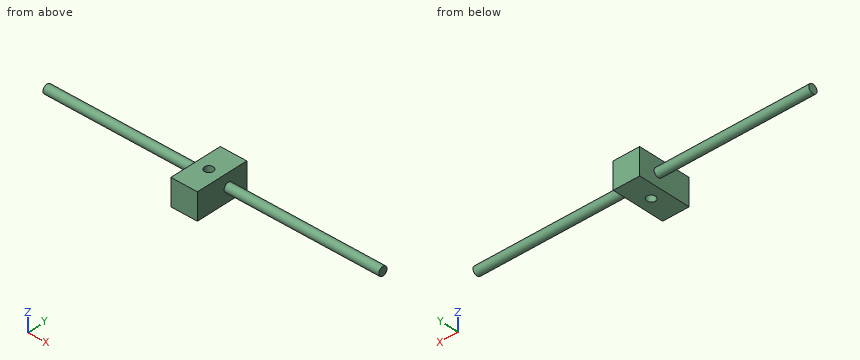
from build123d import *

# Parameters (mm, degrees)
SKETCH_1_W      = 60
SKETCH_1_H      = 120
SKETCH_1_R      = 10
EXTRUDE_1_DEPTH = 30
SKETCH_2_R      = 10
EXTRUDE_2_DEPTH = 350
EXTRUDE_START   = 350
SKETCH_3_R      = 10
EXTRUDE_3_DEPTH = 350


with BuildPart() as part:
    # Эскиз1 → Бобышка-Вытянуть1 (new, symmetric)
    with BuildSketch(Plane.XY):
        Rectangle(SKETCH_1_W, SKETCH_1_H)
        with Locations(Location((0, 0, 0), (0, 0, 180))):
            Circle(SKETCH_1_R, mode=Mode.SUBTRACT)
    extrude(amount=EXTRUDE_1_DEPTH, both=True)

    # Эскиз2 → Бобышка-Вытянуть2 (add)
    with BuildSketch(Plane.ZY.offset(30)):
        with Locations(Location((0, 15, 0), (0, 0, 270))):
            Circle(SKETCH_2_R)
    extrude(amount=EXTRUDE_2_DEPTH)

    # Эскиз3 → Бобышка-Вытянуть3 (add)
    with BuildSketch(Plane(origin=(30, 0, 0), x_dir=(0, 0, -1), z_dir=(1, 0, 0)).offset(EXTRUDE_START)):
        with Locations(Location((0, 15, 0), (0, 0, 270))):
            Circle(SKETCH_3_R)
    extrude(amount=-EXTRUDE_3_DEPTH)


solid = part.part
Can you work these out from the model? Positions are in its coordinate system, mm. Coordinates: 2 decimals unless noted, no trailing zeros. Loops run counter-clockwise (first coordinate to the right, second up) from the corner with the lowest first, then second, coordinate; pieces in that order, holes last. Notation, with made-up numbers: M -40,75.5 L -7,75.5 A23 cw -7,102.5 Z; hole C 14,65 d2. An arc over 180 degrees is marked long. Answer as CSV lines item,"result". Start each with the question number.
1. Suppose I cut it at B-B, the plane x = 0. List the corners of the cut face in (y, z) for me, plus the area to 3 significant figures.
2. Suppose I cut it at C-C, the plane y = -35. List the corners of the cut face in (x, z) for me, plus the area to 3 significant figures.
3. For pin 1 Ø1 at (x, z) = (95, 7.5) entering from -Y; pin 2 Ø10 at (x, z) = (-106.5, -3.5) entering from -Y; pin 3 Ø1.5 at (y, z) = (-15.5, -17) entering from -X, each with a flat end and sliding along its axis, tell me the tip position at first contact or that it passes through.
4. If I drill on probe 1 along Y at (x, z) = (0, -16); probe 2 along X at (y, z) = (49.5, 23); probe 3 along X at (y, z) = (7, -8), over which ranges is the centre line in solid material (lowest first)? Write a range as [from, to].
5. Suppose I cut it at A-A, the plane z = 20.5. List the corners of the cut face in (x, y) for me, plus the area to 3 significant figures.
6. Suppose I cut it at D-D, the plane x = -263.5. List the corners of the cut face in (y, z) for me.
Output:
1,outline,"M -60,-30 L -10,-30 L -10,30 L -60,30 Z; M 10,-30 L 60,-30 L 60,30 L 10,30 Z"
1,area,"6,000 mm^2"
2,outline,"M -30,-30 L 30,-30 L 30,30 L -30,30 Z"
2,area,"3,600 mm^2"
3,pin 1,"stops at y = 7.86"
3,pin 2,"stops at y = 5"
3,pin 3,"stops at x = -30"
4,probe 1,"y = [-60, -10], [10, 60]"
4,probe 2,"x = [-30, 30]"
4,probe 3,"x = [-30, -7.14], [7.14, 30]"
5,outline,"M -30,-60 L 30,-60 L 30,60 L -30,60 Z; hole C 0,0 d20"
5,area,"6,890 mm^2"
6,outline,"C 15,0 d20"
